Could you check a few things on this model? Use its own coordinates, in mm. A direction names the side the tool comes from. Coordinates: 2 decimals unless noted, no trailing zeros. Order: outer loops, then holes, each group sorted by start corner. A loop starts at its lowest first (then second) coordinate and runs counter-clockwise, first axis right, second up. Notation, with made-up numbers: (4.5, 29.25) -> (60.5, 29.25) arc R26 ccw to (60.5, 53.25) -> close; hole circle Ø11 at (18, 67). An arc over 180 degrees is marked (long way). Use a Markdown table: item, result. Add a question column.
1) If I drill on L1, parallel to Y at x = 0, z = 2.5; L2, parallel to Y at x = 0, z = 16; L3, parallel to Z at x = -20, y = 19.5, over which ranges is the centre line in solid material (lowest first)? Write a range as [from, to].
2) Which directions (+Z, -Z, +X, -X, +Y, -Y) give clear straight access to the entire face, cutting with the end or side of a thin tool? Please do faces 1 (the flat face through (13, -6, 5)), 2 (the flat face through (6, 0, -5)).
3) If we section it at D-D (z = 18.75): Write out the boundary of the cut face in (x, y).
4) Will these pins go through, and if not, where does the flat tip stop? pin 1 Ø8 at (x, z) = (11.5, 8) entering from +Y; pin 2 Ø1.5 at (x, y) = (17.5, -2.5) entering from +Z; pin 3 Ø12 at (y, z) = (4.5, 17) entering from +X; pin 4 Ø16 at (x, y) = (0, 0) entering from -Z.
5) If we section it at A-A (y = 0): Write out the boundary of the cut face in (x, z), plus the area to 3 significant figures.
6) If we section it at C-C (z = 0.75): Write out the boundary of the cut face in (x, y).
Autodesk Inventor part; units mm, degrees
ref_plane "YZ Plane" through (0, 0, 0) normal (1, 0, 0) x (0, 1, 0)
ref_plane "XZ Plane" through (0, 0, 0) normal (0, 1, 0) x (-1, 0, 0)
ref_plane "XY Plane" through (0, 0, 0) normal (0, 0, 1) x (1, 0, 0)
sketch "Sketch1" plane through (0, 0, 0) normal (0, 0, 1) x (1, 0, 0)
  circle A0 centre (0, 0) radius 30
  dimension "d0" = 60
extrude "Extrusion1" add sketch "Sketch1" along normal mid plane 10
sketch "Sketch2" plane through (0, 0, 5) normal (0, 0, 1) x (1, 0, 0)
  circle A0 centre (0, 0) radius 30
  circle A1 centre (0, 0) radius 10
  dimension "d3" = 20
extrude "Extrusion2" add sketch "Sketch2" along normal blind 20 contours A1
sketch "Sketch3" plane through (0, 0, 25) normal (0, 0, 1) x (1, 0, 0)
  circle A0 centre (0, 0) radius 10
  circle A1 centre (0, 0) radius 5
  dimension "d6" = 10
extrude "Extrusion3" cut sketch "Sketch3" against normal through all contours A1
fillet "Fillet1" radius 3 1 edges at (-10, 0, 5)
chamfer "Chamfer1" distance 1 angle 45 1 edges at (-10, 0, 25)
sketch "Sketch5" plane through (0, 0, 5) normal (0, 0, 1) x (1, 0, 0)
  circle A0 centre (0, 0) radius 30
  circle A1 centre (0, 0) radius 5
  point P0 (-21, 0)
  point P1 (21, 0)
  point P2 (0, 21)
  point P3 (0, -21)
  dimension "d14" = 21
  dimension "d15" = 21
  dimension "d16" = 21
  dimension "d17" = 21
hole "Hole1" at (-21, 0, 5) at (21, 0, 5) at (0, 21, 5) at (0, -21, 5) direction (0, 0, -1) diameter 3 end through all
chamfer "Chamfer2" distance 0.5 angle 45 1 edges at (-30, 0, 5)
properties part number "relation"
Answer sheet:
| question | item | result |
|---|---|---|
| 1 | L1 | [-30, -22.5], [-19.5, -5], [5, 19.5], [22.5, 30] |
| 1 | L2 | [-10, -5], [5, 10] |
| 1 | L3 | [-5, 5] |
| 2 | face 1 | +Z |
| 2 | face 2 | -Z, +X, -X, +Y, -Y |
| 3 | outline | circle Ø20 at (0, 0); hole circle Ø10 at (0, 0) |
| 4 | pin 1 | y = 28.43 |
| 4 | pin 2 | z = 5 |
| 4 | pin 3 | x = 10 |
| 4 | pin 4 | z = -5 |
| 5 | outline | (-30, -5) -> (-22.5, -5) -> (-22.5, 5) -> (-29.5, 5) -> (-30, 4.5) -> close; (-19.5, -5) -> (-5, -5) -> (-5, 25) -> (-9, 25) -> (-10, 24) -> (-10, 8) arc R3 cw to (-13, 5) -> (-19.5, 5) -> close; (5, -5) -> (19.5, -5) -> (19.5, 5) -> (13, 5) arc R3 cw to (10, 8) -> (10, 24) -> (9, 25) -> (5, 25) -> close; (22.5, -5) -> (30, -5) -> (30, 4.5) -> (29.5, 5) -> (22.5, 5) -> close |
| 5 | area | 643 mm2 |
| 6 | outline | circle Ø60 at (0, 0); hole circle Ø3 at (-21, 0); hole circle Ø10 at (0, 0); hole circle Ø3 at (0, -21); hole circle Ø3 at (0, 21); hole circle Ø3 at (21, 0) |
